For this review, take the finished solid that the model builds, in its own axes (mm). Face numbers are marked on the shaded views. Give positions to 0.01 mm unless a question says otherwise; leave off trailing zeros. Write each loop counter-clockwise with the first axis right and the second up, starting at its lowest first coordinate (ties: lowest second). Pieces come first, ordered by that corner, then holes. Notation, with made-up numbers: M 60.5,-19 L 119.5,-19 A7 cw 119.5,-15 Z; hole C 56,37.5 d10. An arc over 180 degrees is marked long. One line per item, written item: value. Start each with the question number.
Item 1: To check wall thickness, follow probe 1 along X at (y, z) = (5, 2.05); probe 2 along Y at (x, z) = (0, 0.7); probe 3 along X at (y, z) = (2, 2.2). State the ranges of each line that lie inside material, in increasing order.
Item 2: Consider section A-A, the plane x = 0. Write out the cut boundary in (y, z), and give its area (3 significant figures).
Item 3: Consider section B-B, the plane z = 0.75. Write out the cut boundary in (x, y).
Item 4: Mouldability with a two-part tool opening along Y and no side actions: class the marked faces 1, 2, 3 and 4 as released by +Y, released by -Y, zero draft, split by the parting line, or undercut.
Item 5: Clearance check with flat-ended pins moving along their axes: pin 1 Ø1 at (y, z) = (-13, 1) entering from -X; pin 2 Ø1.5 at (x, z) = (-7.5, 1) entering from -Y. State where each tip first meets the part, or that it passes through.
```python
from build123d import *

# Parameters (mm, degrees)
F0_R         = 4.1761867796
F0_R_2       = 4.3460448691
F1_DEPTH     = 2.54
F2_DEPTH     = 12.7
F3_R         = 7.2200461369
F4_DEPTH     = 12.7
F7_T1_DEPTH  = 14.697191958
F7_T3_DEPTH  = 10.4099383433
F7_T5_DEPTH  = 30.8011159773
F7_T7_DEPTH  = 35.5510768625
F7_T9_DEPTH  = 17.7553157696
F7_T11_DEPTH = 18.6111496066
F7_T14_ANGLE = 198.1944914786
F7_T23_DEPTH = 17.7553157696
F7_T27_DEPTH = 18.6111496066


# Not quite as in the source:
# - a fillet or chamfer that OpenCascade refuses, or shapes differently, is made with other operations: its cross-section is extruded or revolved along the edge and cut away or added


with BuildPart() as f1:
    # F0 (on Top) → F1 (new body)
    with BuildSketch(Plane.XY):
        Polygon((-16.1636956036, 7.9843616113), (-16.1636956036, 0), (-16.1636956036, -3.5330012906), (0.857539475, -3.5330012906), (0.857539475, -6.9984025322), (16.9614627957, -6.9984025322), (16.9614627957, 0), (16.9614627957, 12.6728452742), (-10.6598241255, 12.6728452742), align=None)
        with Locations((-10.1569462568, 4.5435167849)):
            Circle(F0_R, mode=Mode.SUBTRACT)
        with Locations((0, 5.0288974307)):
            Circle(F0_R_2, mode=Mode.SUBTRACT)
    extrude(amount=F1_DEPTH)

    # F2 (add): a face of the model
    f2_faces = [f1.faces().sort_by_distance(p)[0] for p in [
        (8.9095011353, -6.9984025322, 1.27),
    ]]
    extrude(f2_faces, amount=F2_DEPTH)


with BuildPart() as f4:
    # F3 (on Top) → F4 (new body)
    with BuildSketch(Plane.XY):
        with Locations((6.5507800318, -27.7640167624)):
            Circle(F3_R)
    extrude(amount=F4_DEPTH)


with BuildPart() as f4_1:
    # F5: moved
    add(f4.part.moved(Location((2.54, 7.62, 0))))


with BuildPart() as f1_1:
    add(f1.part)

    # F6: cut F4
    add(f4_1.part, mode=Mode.SUBTRACT)

    # F7: fillet of radius 0.635 on 11 edges, made by hand

    # F7_s2 → F7_t1 (cut)
    with BuildSketch(Plane.XZ.offset(-9.5742761394)):
        with BuildLine():
            ThreePointArc((-16.1640956036, 1.9040343146), (-15.9777084097, 2.3540128061), (-15.5277299182, 2.5404))
            Line((-15.5277299182, 2.5404), (-15.5277299182, 2.6040365685))
            ThreePointArc((-15.5277299182, 2.6040365685), (-15.8457127609, 2.6036365685), (-16.1636956036, 2.6036365685))
            Line((-16.1636956036, 2.6036365685), (-16.2273321722, 2.54))
            ThreePointArc((-16.2273321722, 2.54), (-16.2273321722, 2.2220171573), (-16.2277321722, 1.9040343146))
            Line((-16.2277321722, 1.9040343146), (-16.1640956036, 1.9040343146))
        make_face()
    extrude(amount=F7_T1_DEPTH, mode=Mode.SUBTRACT)

    # F7_s4 → F7_t3 (cut)
    with BuildSketch(Plane(origin=(1.2888696755, 1.0979261491, 0), x_dir=(0, 0, 1), z_dir=(-0.7612431928, -0.6484664998, 0))):
        with BuildLine():
            ThreePointArc((1.9040343146, 16.560056038), (2.3540128061, 16.373668844), (2.5404, 15.9236903525))
            Line((2.5404, 15.9236903525), (2.6040365685, 15.9236903525))
            ThreePointArc((2.6040365685, 15.9236903525), (2.6036365685, 16.2416731952), (2.6036365685, 16.559656038))
            Line((2.6036365685, 16.559656038), (2.54, 16.6232926065))
            ThreePointArc((2.54, 16.6232926065), (2.2220171573, 16.6232926065), (1.9040343146, 16.6236926065))
            Line((1.9040343146, 16.6236926065), (1.9040343146, 16.560056038))
        make_face()
    extrude(amount=F7_T3_DEPTH, mode=Mode.SUBTRACT)

    # F7_s6 → F7_t5 (cut)
    with BuildSketch(Plane.YZ.offset(-12.2497386535)):
        with BuildLine():
            ThreePointArc((12.0368795888, 2.5404), (12.4868580803, 2.3540128061), (12.6732452742, 1.9040343146))
            Line((12.6732452742, 1.9040343146), (12.7368818428, 1.9040343146))
            ThreePointArc((12.7368818428, 1.9040343146), (12.7364818428, 2.2220171573), (12.7364818428, 2.54))
            Line((12.7364818428, 2.54), (12.6728452742, 2.6036365685))
            ThreePointArc((12.6728452742, 2.6036365685), (12.3548624315, 2.6036365685), (12.0368795888, 2.6040365685))
            Line((12.0368795888, 2.6040365685), (12.0368795888, 2.5404))
        make_face()
    extrude(amount=F7_T5_DEPTH, mode=Mode.SUBTRACT)

    # F7_s8 → F7_t7 (cut)
    with BuildSketch(Plane.XZ.offset(-14.2627598023)):
        with BuildLine():
            ThreePointArc((16.3254971103, 2.5404), (16.7754756018, 2.3540128061), (16.9618627957, 1.9040343146))
            Line((16.9618627957, 1.9040343146), (17.0254993643, 1.9040343146))
            ThreePointArc((17.0254993643, 1.9040343146), (17.0250993643, 2.2220171573), (17.0250993643, 2.54))
            Line((17.0250993643, 2.54), (16.9614627957, 2.6036365685))
            ThreePointArc((16.9614627957, 2.6036365685), (16.643479953, 2.6036365685), (16.3254971103, 2.6040365685))
            Line((16.3254971103, 2.6040365685), (16.3254971103, 2.5404))
        make_face()
    extrude(amount=F7_T7_DEPTH, mode=Mode.SUBTRACT)

    # F7_s10 → F7_t9 (cut)
    with BuildSketch(Plane.XZ.offset(3.5330012906)):
        with BuildLine():
            ThreePointArc((1.4935051604, 2.5404), (1.0435266689, 2.3540128061), (0.857139475, 1.9040343146))
            Line((0.857139475, 1.9040343146), (0.7935029064, 1.9040343146))
            ThreePointArc((0.7935029064, 1.9040343146), (0.7939029064, 2.2220171573), (0.7939029064, 2.54))
            Line((0.7939029064, 2.54), (0.857539475, 2.6036365685))
            ThreePointArc((0.857539475, 2.6036365685), (1.1755223177, 2.6036365685), (1.4935051604, 2.6040365685))
            Line((1.4935051604, 2.6040365685), (1.4935051604, 2.5404))
        make_face()
    extrude(amount=F7_T9_DEPTH, mode=Mode.SUBTRACT)

    # F7_s12 → F7_t11 (cut)
    with BuildSketch(Plane.YZ.offset(-17.7536101317)):
        with BuildLine():
            ThreePointArc((-2.8970356052, 2.5404), (-3.3470140967, 2.3540128061), (-3.5334012906, 1.9040343146))
            Line((-3.5334012906, 1.9040343146), (-3.5970378592, 1.9040343146))
            ThreePointArc((-3.5970378592, 1.9040343146), (-3.5966378592, 2.2220171573), (-3.5966378592, 2.54))
            Line((-3.5966378592, 2.54), (-3.5330012906, 2.6036365685))
            ThreePointArc((-3.5330012906, 2.6036365685), (-3.2150184479, 2.6036365685), (-2.8970356052, 2.6040365685))
            Line((-2.8970356052, 2.6040365685), (-2.8970356052, 2.5404))
        make_face()
    extrude(amount=F7_T11_DEPTH, mode=Mode.SUBTRACT)

    # F7_s13 → F7_t14 (revolve, cut)
    with BuildSketch(Plane(origin=(3.3721800717, -21.0597061225, 0), x_dir=(0, 0, 1), z_dir=(0.1581106012, -0.9874214084, 0))):
        with BuildLine():
            ThreePointArc((2.5404, 2.0645636003), (2.3540128061, 1.6145851088), (1.9040343146, 1.4281979149))
            Line((1.9040343146, 1.4281979149), (1.9040343146, 1.3645613463))
            ThreePointArc((1.9040343146, 1.3645613463), (2.2220171573, 1.3649613463), (2.54, 1.3649613463))
            Line((2.54, 1.3649613463), (2.6036365685, 1.4285979149))
            ThreePointArc((2.6036365685, 1.4285979149), (2.6036365685, 1.7465807576), (2.6040365685, 2.0645636003))
            Line((2.6040365685, 2.0645636003), (2.5404, 2.0645636003))
        make_face()
    revolve(axis=Axis((9.0907800318, -20.1440167624, 2.54), (0, 0, -1)), revolution_arc=F7_T14_ANGLE, mode=Mode.SUBTRACT)

    # F7_s15 → F7_t16 (revolve, cut)
    with BuildSketch(Plane.XZ.offset(-4.5435167849)):
        with BuildLine():
            ThreePointArc((-5.3447937917, 2.5404), (-5.7947722832, 2.3540128061), (-5.9811594771, 1.9040343146))
            Line((-5.9811594771, 1.9040343146), (-6.0447960457, 1.9040343146))
            ThreePointArc((-6.0447960457, 1.9040343146), (-6.0443960457, 2.2220171573), (-6.0443960457, 2.54))
            Line((-6.0443960457, 2.54), (-5.9807594771, 2.6036365685))
            ThreePointArc((-5.9807594771, 2.6036365685), (-5.6627766344, 2.6036365685), (-5.3447937917, 2.6040365685))
            Line((-5.3447937917, 2.6040365685), (-5.3447937917, 2.5404))
        make_face()
    revolve(axis=Axis((-10.1569462568, 4.5435167849, 2.54), (0, 0, 1)), mode=Mode.SUBTRACT)

    # F7_s17 → F7_t18 (revolve, cut)
    with BuildSketch(Plane.XZ.offset(-5.0288974307)):
        with BuildLine():
            ThreePointArc((4.9820105545, 2.5404), (4.532032063, 2.3540128061), (4.3456448691, 1.9040343146))
            Line((4.3456448691, 1.9040343146), (4.2820083005, 1.9040343146))
            ThreePointArc((4.2820083005, 1.9040343146), (4.2824083005, 2.2220171573), (4.2824083005, 2.54))
            Line((4.2824083005, 2.54), (4.3460448691, 2.6036365685))
            ThreePointArc((4.3460448691, 2.6036365685), (4.6640277118, 2.6036365685), (4.9820105545, 2.6040365685))
            Line((4.9820105545, 2.6040365685), (4.9820105545, 2.5404))
        make_face()
    revolve(axis=Axis((0, 5.0288974307, 2.54), (0, 0, 1)), mode=Mode.SUBTRACT)


with BuildPart() as f7_tool21:
    # F7_s22 → F7_t23 (new body)
    with BuildSketch(Plane.XZ.offset(1.9430867626)):
        with BuildLine():
            ThreePointArc((1.4935051604, 2.5404), (1.0435266689, 2.3540128061), (0.857139475, 1.9040343146))
            Line((0.857139475, 1.9040343146), (0.7935029064, 1.9040343146))
            ThreePointArc((0.7935029064, 1.9040343146), (0.7939029064, 2.2220171573), (0.7939029064, 2.54))
            Line((0.7939029064, 2.54), (0.857539475, 2.6036365685))
            ThreePointArc((0.857539475, 2.6036365685), (1.1755223177, 2.6036365685), (1.4935051604, 2.6040365685))
            Line((1.4935051604, 2.6040365685), (1.4935051604, 2.5404))
        make_face()
    extrude(amount=F7_T23_DEPTH)

    split(bisect_by=Plane.XZ.offset(3.5330012906), keep=Keep.BOTTOM)


with BuildPart() as f7_tool25:
    # F7_s26 → F7_t27 (new body)
    with BuildSketch(Plane.YZ.offset(-16.1636956036)):
        with BuildLine():
            ThreePointArc((-2.8970356052, 2.5404), (-3.3470140967, 2.3540128061), (-3.5334012906, 1.9040343146))
            Line((-3.5334012906, 1.9040343146), (-3.5970378592, 1.9040343146))
            ThreePointArc((-3.5970378592, 1.9040343146), (-3.5966378592, 2.2220171573), (-3.5966378592, 2.54))
            Line((-3.5966378592, 2.54), (-3.5330012906, 2.6036365685))
            ThreePointArc((-3.5330012906, 2.6036365685), (-3.2150184479, 2.6036365685), (-2.8970356052, 2.6040365685))
            Line((-2.8970356052, 2.6040365685), (-2.8970356052, 2.5404))
        make_face()
    extrude(amount=F7_T27_DEPTH)

    split(bisect_by=Plane.YZ.offset(0.857539475), keep=Keep.TOP)


with BuildPart() as f7_tool21_1:
    add(f7_tool21.part)

    # F7_t29: intersect F7_tool25
    add(f7_tool25.part, mode=Mode.INTERSECT)


with BuildPart() as f1_2:
    add(f1_1.part)

    # F7_t19: cut F7_tool21
    add(f7_tool21_1.part, mode=Mode.SUBTRACT)


solid = f1_2.part
```
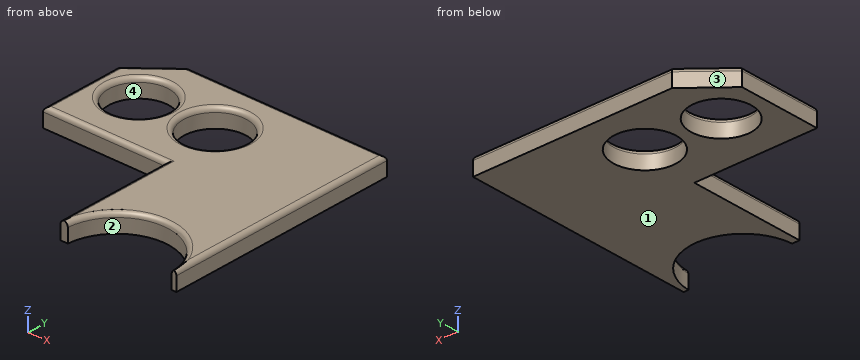
Model answer:
1. probe 1: x = -16.15 to -14.32, -5.99 to -4.36, 4.36 to 16.94
1. probe 2: y = -3.53 to 0.68, 9.37 to 12.67
1. probe 3: x = -16.09 to -13.56, -6.75 to -3.22, 3.22 to 16.89
2. outline: M -3.53,0 L 0.68,0 L 0.68,1.93 A0.64 ccw 0.07,2.54 L -2.92,2.54 A0.64 ccw -3.53,1.93 Z; M 9.37,0 L 12.67,0 L 12.67,1.93 A0.64 ccw 12.06,2.54 L 9.99,2.54 A0.64 ccw 9.37,1.93 Z
2. area: 18.7 mm2
3. outline: M -16.16,-3.53 L 0.86,-3.53 L 0.86,-19.7 L 1.88,-19.7 A7.22 cw 16.3,-19.7 L 16.96,-19.7 L 16.96,12.67 L -10.66,12.67 L -16.16,7.98 Z; hole C -10.16,4.54 d8.35; hole C 0,5.03 d8.69
4. face 1: zero draft
4. face 2: released by -Y
4. face 3: released by +Y
4. face 4: undercut
5. pin 1: stops at x = 0.86
5. pin 2: stops at y = -3.53
